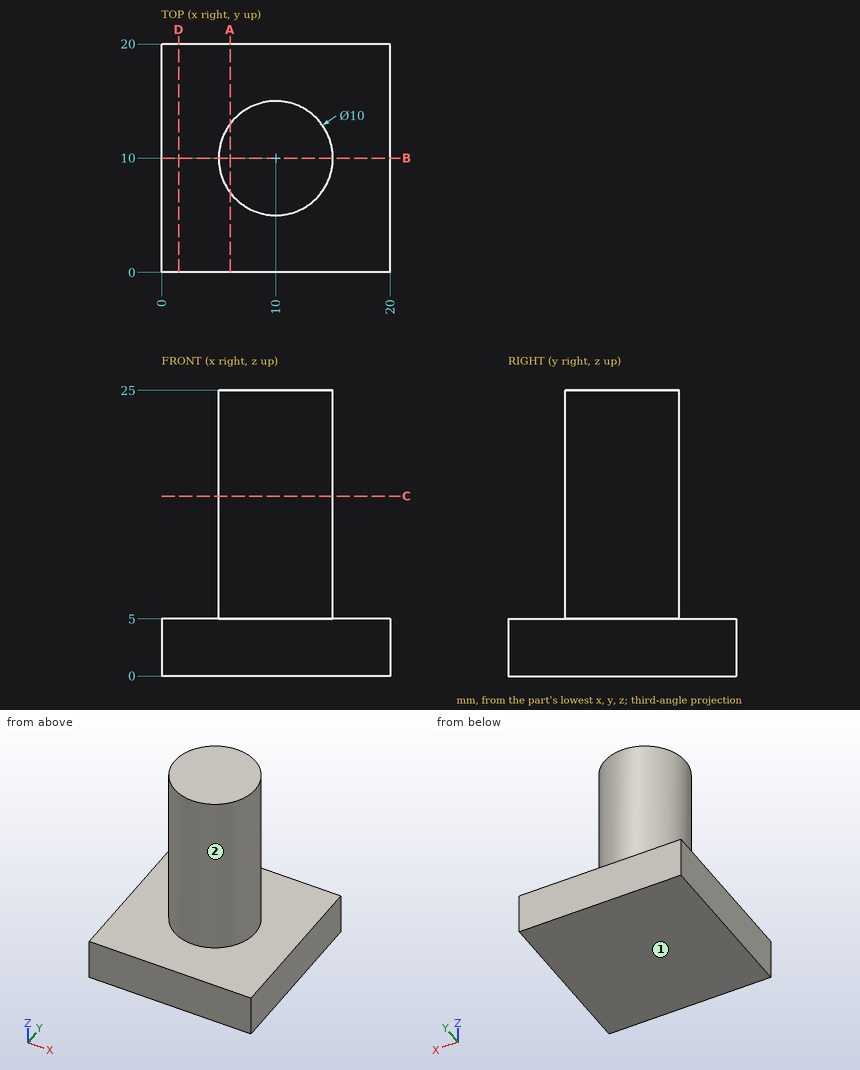
Study the drawing (mm; zero at the part's minimum x, y, z) and answer. A direction names the side the tool comes from. Round coordinates to 2 decimals unless told otherwise and drop trailing zeros. Write each loop counter-clockwise with the first axis right and the second up, starting at its lowest first coordinate (ties: lowest second). Pieces come first, ordered by that corner, then holes. Notation, with made-up numbers: (88, -23.5) - (94, -23.5) arc R24 ccw to (94, -11.5) - close; hole circle Ø3 at (-19.75, 68.5). An arc over 180 degrees is marked (long way). Use a Markdown table: item, result. Add a question column.
1. The part is cut by section C-C (z = 15.75). Write down the section's boundary in (x, y), and give its area (3 significant figures).
2. Consider line 1 (X direction, y = 9.75, z = 17.75); line 2 (Z direction, x = 2, y = 3.5). Determine where each line is inside the solid, lowest interval first.
3. A tool of negligible diameter and unlimited length cuts with its end or side. For the marked faces 1 and 2, from which of +Z, -Z, +X, -X, +Y, -Y can it reach the whole face along a straight path? Write none if from no direction.
4. The part is cut by section A-A (x = 6). Write down the section's boundary in (y, z).
5. Flat-ended cylindrical pins translate along their axes: P1, Ø2, axis at x = 2, y = 6, coming from the +Z side; P2, Ø3, axis at x = 14, z = 17.5, coming from the -Y side; P3, Ø2, axis at x = 9, z = 15.5, coming from the -Y side. Find the tip coordinate at first contact, or state that the pin passes through.
6. The part is cut by section D-D (x = 1.5). Write down the section's boundary in (y, z), and give its area (3 significant figures).
7. The part is cut by section B-B (y = 10). Write down the section's boundary in (x, z).
Reported:
| question | item | result |
|---|---|---|
| 1 | outline | circle Ø10 at (10, 10) |
| 1 | area | 78.5 mm^2 |
| 2 | line 1 | 5.01 to 14.99 |
| 2 | line 2 | 0 to 5 |
| 3 | face 1 | -Z, +X, -X, +Y, -Y |
| 3 | face 2 | +Z |
| 4 | outline | (0, 0) - (20, 0) - (20, 5) - (13, 5) - (13, 25) - (7, 25) - (7, 5) - (0, 5) - close |
| 5 | P1 | z = 5 |
| 5 | P2 | y = 5.67 |
| 5 | P3 | y = 5 |
| 6 | outline | (0, 0) - (20, 0) - (20, 5) - (0, 5) - close |
| 6 | area | 100 mm^2 |
| 7 | outline | (0, 0) - (20, 0) - (20, 5) - (15, 5) - (15, 25) - (5, 25) - (5, 5) - (0, 5) - close |
